Geometry: final body of the model. Coordinates: model frame, mm. A direction names the side the tool comes from. Round coordinates to 2 decimals unless told otherwise and drop trailing zeros. Write each loop counter-clockwise with the first axis right and the second up, starting at its lowest first coordinate (ties: lowest second). Pieces come first, ordered by that corner, then holes. Notation, with made-up numbers: M 66,11.5 L 124,11.5 A12 cw 124,20.5 Z; hole C 83.5,-19 d7. An arc over 180 degrees is marked long. Use one line per item in the form item = value. Start each with the question number.
Item 1: Section query B-B (y = 18). Return loops of the section in (x, z).
Item 2: Pin query (flat end, axial travel): pin 1 Ø4 at (y, z) = (20.5, 12) entering from +X; pin 2 Ø3.5 at (x, y) = (-48, 4) entering from +Z; pin 3 Ø12 at (y, z) = (14, 17.5) entering from +X. Return the tip coordinate at first contact, or that it passes through.
Item 3: Section query C-C (z = 12). Return loops of the section in (x, y), and give its area (3 significant figures).
Item 4: Ray query, probe 1 along X at (y, z) = (6, 9.5); probe 2 along X at (y, z) = (14.5, 14); probe 3 along Y at (x, z) = (-22.5, -0.5). Return the intervals inside material, ascending.
Item 5: Section query A-A (x = -48.4). Return loops of the section in (y, z) (3 decimals).
Item 6: Section query D-D (y = 31.75). Return loops of the section in (x, z).
Item 7: Pull-direction query (X, two-part tool) for faces 1 (the flat face through (-5.1, 4.479, -2.155)), 2 (the flat face through (-1.5, 22, -6)), 3 (the flat face through (-15, 0, 2)); classes: pulls with the +X half, pulls with the -X half, needs draft (parallel to the pull), parting line crosses it, or undercut.
Item 8: Reachability of faces 4 (the flat face through (-48, 4, -0.125)), 5 (the cylindrical face through (-4.17, 4.521, -6.524)), 6 (the flat face through (-37, 1, 0)), 7 (the flat face through (0, 1, -4)), 8 (the flat face through (-48, 4, -6.525)) from +Z, -Z, +X, -X, +Y, -Y: full face, straight path, thin tool, end or side. Return the list, or none.
from build123d import *

# Parameters (mm, degrees)
SKETCH1_W               = 56
SKETCH1_H               = 7.25
SKETCH1_R               = 1.6
SKETCH1_W_2             = 5
SKETCH1_H_2             = 16.75
SKETCH1_W_3             = 11.5
BOSS_EXTRUDE1_DEPTH     = 3
SKETCH2_W               = 8
SKETCH2_H               = 7
BOSS_EXTRUDE2_DEPTH     = 3
FILLET1_R               = 2
SKETCH3_W               = 16
SKETCH3_H               = 16
BOSS_EXTRUDE3_DEPTH     = 4
BOSS_EXTRUDE4_DEPTH     = 3
BOSS_EXTRUDE5_DEPTH     = 2
BOSS_EXTRUDE6_DEPTH     = 2
CHAMFER1_SIZE           = 3
SKETCH8_W               = 8
SKETCH8_H               = 10
CUT_EXTRUDE1_DEPTH      = 10
CUT_EXTRUDE2_DEPTH      = 74.518705103
CUT_EXTRUDE2_DEPTH_BACK = 2
CUT_EXTRUDE3_DEPTH      = 72.281133549
CUT_EXTRUDE3_DEPTH_BACK = 2
SKETCH11_R              = 1.5
BOSS_EXTRUDE7_DEPTH     = 3
SKETCH13_R              = 2.5
BOSS_EXTRUDE8_DEPTH     = 1.5


with BuildPart() as part:
    # Sketch1 → Boss-Extrude1 (new body)
    # profile 1 of 4: a face of its own
    with BuildSketch(Plane(origin=(0, 0, 0), x_dir=(1, 0, 0), z_dir=(0, 1, 0))):
        with Locations((-28, 3.625)):
            Rectangle(SKETCH1_W, SKETCH1_H)
        with Locations(Location((-7.6, 3.625, 0), (0, 0, 270))):
            Circle(SKETCH1_R, mode=Mode.SUBTRACT)
        with Locations(Location((-48.4, 3.625, 0), (0, 0, 270))):
            Circle(SKETCH1_R, mode=Mode.SUBTRACT)
    # profile 2 of 4: a face of its own
    with BuildSketch(Plane(origin=(0, 0, 0), x_dir=(1, 0, 0), z_dir=(0, 1, 0))):
        with Locations((-2.5, -8.375)):
            Rectangle(SKETCH1_W_2, SKETCH1_H_2)
    # profile 3 of 4: a face of its own
    with BuildSketch(Plane(origin=(0, 0, 0), x_dir=(1, 0, 0), z_dir=(0, 1, 0))):
        with Locations((5.75, -8.375)):
            Rectangle(SKETCH1_W_3, SKETCH1_H_2)
    # profile 4 of 4: a face of its own
    with BuildSketch(Plane(origin=(0, 0, 0), x_dir=(1, 0, 0), z_dir=(0, 1, 0))):
        with Locations((-10.75, -8.375)):
            Rectangle(SKETCH1_W_3, SKETCH1_H_2)
    extrude(amount=BOSS_EXTRUDE1_DEPTH)

    # Sketch2 → Boss-Extrude2 (add)
    # profile 1 of 2: a face of its own
    with BuildSketch(Plane(origin=(0, 3, 0), x_dir=(1, 0, 0), z_dir=(0, 1, 0))):
        with Locations((-48.4, 3.625)):
            Rectangle(SKETCH2_W, SKETCH2_H)
        Polygon((-46.725684219, 0.725), (-45.051368439, 3.625), (-46.725684219, 6.525), (-50.074315781, 6.525), (-51.748631561, 3.625), (-50.074315781, 0.725), align=None, mode=Mode.SUBTRACT)
    # profile 2 of 2: a face of its own
    with BuildSketch(Plane(origin=(0, 3, 0), x_dir=(1, 0, 0), z_dir=(0, 1, 0))):
        with Locations((-7.6, 3.625)):
            Rectangle(SKETCH2_W, SKETCH2_H)
        Polygon((-5.925684219, 0.725), (-4.251368439, 3.625), (-5.925684219, 6.525), (-9.274315781, 6.525), (-10.948631561, 3.625), (-9.274315781, 0.725), align=None, mode=Mode.SUBTRACT)
    extrude(amount=BOSS_EXTRUDE2_DEPTH)

    # Fillet1
    fillet1_edges = [part.edges().sort_by_distance(p)[0] for p in [
        (-44.4, 4.5, -0.125),
        (-44.4, 4.5, -7.125),
        (-52.4, 4.5, -7.125),
        (-52.4, 4.5, -0.125),
        (-3.6, 4.5, -0.125),
        (-3.6, 4.5, -7.125),
        (-11.6, 4.5, -7.125),
        (-11.6, 4.5, -0.125),
    ]]
    fillet(fillet1_edges, radius=FILLET1_R)

    # Sketch3 → Boss-Extrude3 (add)
    with BuildSketch(Plane(origin=(0, 3, 0), x_dir=(1, 0, 0), z_dir=(0, 1, 0))):
        with Locations((3.5, -8.75)):
            Rectangle(SKETCH3_W, SKETCH3_H)
    extrude(amount=BOSS_EXTRUDE3_DEPTH)

    # Sketch5 → Boss-Extrude4 (add)
    with BuildSketch(Plane.ZY.offset(4.5)):
        Polygon((-13.25, 7), (0.75, 7), (16.75, 7), (26.75, 7), (26.75, 37), (-13.25, 37), align=None)
    extrude(amount=-BOSS_EXTRUDE4_DEPTH)

    # Sketch6 → Boss-Extrude5 (add)
    with BuildSketch(Plane.XY.offset(16.75)):
        Polygon((-1.5, 37), (0, 37), (11.5, 7), (-1.5, 7), align=None)
    extrude(amount=-BOSS_EXTRUDE5_DEPTH)

    # Sketch7 → Boss-Extrude6 (add)
    with BuildSketch(Plane(origin=(0, 0, 0.75), x_dir=(-1, 0, 0), z_dir=(0, 0, -1))):
        Polygon((1.5, 37), (0, 37), (-11.5, 7), (1.5, 7), align=None)
    extrude(amount=-BOSS_EXTRUDE6_DEPTH)

    # Chamfer1
    chamfer1_edges = [part.edges().sort_by_distance(p)[0] for p in [
        (-3, 7, -13.25),
        (-3, 37, -13.25),
        (-3, 37, 26.75),
        (-3, 7, 26.75),
    ]]
    chamfer(chamfer1_edges, length=CHAMFER1_SIZE)

    # Sketch8 → Cut-Extrude1 (cut)
    with BuildSketch(Plane(origin=(-1.5, 0, 0), x_dir=(0, 0, -1), z_dir=(1, 0, 0))):
        with Locations((-8.75, 22)):
            Rectangle(SKETCH8_W, SKETCH8_H)
    extrude(amount=-CUT_EXTRUDE1_DEPTH, mode=Mode.SUBTRACT)

    # Sketch9 → Cut-Extrude2 (cut, two sides: drawn at the far end of the back side and taken through both)
    with BuildSketch(Plane.XY.offset(16.75).offset(-CUT_EXTRUDE2_DEPTH_BACK)):
        Polygon((0, 185.220530074), (0, 37), (0, 13.52173913), (9, 13.52173913), (157.220530074, 13.52173913), (375.851096448, 213.716588185), (218.630566375, 385.415379128), align=None)
    extrude(amount=CUT_EXTRUDE2_DEPTH + CUT_EXTRUDE2_DEPTH_BACK, mode=Mode.SUBTRACT)

    # Sketch10 → Cut-Extrude3 (cut, two sides: drawn at the far end of the back side and taken through both)
    with BuildSketch(Plane.XY.offset(2.75).offset(-CUT_EXTRUDE3_DEPTH_BACK)):
        Polygon((0, 185.220530074), (0, 37), (0, 13.52173913), (9, 13.52173913), (157.220530074, 13.52173913), (375.851096448, 213.716588185), (218.630566375, 385.415379128), align=None)
    extrude(amount=CUT_EXTRUDE3_DEPTH + CUT_EXTRUDE3_DEPTH_BACK, mode=Mode.SUBTRACT)

    # Sketch11 → Boss-Extrude7 (add)
    with BuildSketch(Plane(origin=(-1.5, 0, 0), x_dir=(0, 0, -1), z_dir=(1, 0, 0))):
        with Locations(Location((-8.75, 31.75, 0), (0, 0, 180))):
            Circle(SKETCH11_R)
        with Locations(Location((-8.75, 12.25, 0), (0, 0, 180))):
            Circle(SKETCH11_R)
    extrude(amount=BOSS_EXTRUDE7_DEPTH)

    # Sketch13 → Boss-Extrude8 (add)
    with BuildSketch(Plane(origin=(-1.5, 0, 0), x_dir=(0, 0, -1), z_dir=(1, 0, 0))):
        with Locations(Location((-8.75, 31.75, 0), (0, 0, 180))):
            Circle(SKETCH13_R)
        with Locations(Location((-8.75, 12.25, 0), (0, 0, 180))):
            Circle(SKETCH13_R)
    extrude(amount=BOSS_EXTRUDE8_DEPTH)


solid = part.part
Working result:
q1.outline = M -4.5,-13.25 L -1.5,-13.25 L -1.5,0.75 L 0,0.75 L 0,2.75 L -1.5,2.75 L -1.5,4.75 L -4.5,4.75 Z; M -4.5,12.75 L -1.5,12.75 L -1.5,14.75 L 0,14.75 L 0,16.75 L -1.5,16.75 L -1.5,26.75 L -4.5,26.75 Z
q2.pin_1 = -1.5
q2.pin_2 = 0
q2.pin_3 = 11.1
q3.outline = M -16.5,0 L 11.5,0 L 11.5,7 L -1.5,7 L -1.5,17 L -4.5,17 L -4.5,3 L -16.5,3 Z; M -4.5,27 L -1.5,27 L -1.5,37 L -4.5,37 Z
q3.area = 208 mm²
q4.probe_1 = -4.5 to 11.5
q4.probe_2 = -4.5 to -1.5
q4.probe_3 = 0 to 3
q5.outline = M 0,-7.25 L 3,-7.25 L 3,-7.125 L 6,-7.125 L 6,-6.525 L 3,-6.525 L 3,-5.225 L 0,-5.225 Z; M 0,-2.025 L 3,-2.025 L 3,-0.725 L 6,-0.725 L 6,-0.125 L 3,-0.125 L 3,0 L 0,0 Z
q6.outline = M -4.5,-13.25 L -1.5,-13.25 L -1.5,0.75 L 0,0.75 L 0,2.75 L -1.5,2.75 L -1.5,6.25 L 0,6.25 L 0,7.25 L 1.5,7.25 L 1.5,10.25 L 0,10.25 L 0,11.25 L -1.5,11.25 L -1.5,14.75 L 0,14.75 L 0,16.75 L -1.5,16.75 L -1.5,26.75 L -4.5,26.75 Z
q7.face_1 = undercut
q7.face_2 = pulls with the +X half
q7.face_3 = needs draft
q8.face_4 = +Z, +X, -X, +Y
q8.face_5 = -Z, +X
q8.face_6 = +Z, -X, +Y, -Y
q8.face_7 = -Z, +X, +Y, -Y
q8.face_8 = +Y
